```python
from build123d import *

# Parameters (mm, degrees)
PAD002_DEPTH    = 3
SKETCH008_R     = 1.5
SKETCH008_W     = 3
SKETCH008_H     = 26
POCKET001_DEPTH = 3.001
POCKET002_DEPTH = 3.001
SKETCH011_R     = 2.25
HOLE003_DEPTH   = 3.001


with BuildPart() as part:
    # Sketch005 → Pad002 (new body)
    with BuildSketch(Plane.XZ):
        Polygon((-30, 0), (-30, 70), (50, 70), (50, 0), (25, 0), (25, 5.5), (26.5, 5.5), (26.5, 10), (20.5, 10), (20.5, 5.5), (22, 5.5), (22, 0), (20.5, 0), (20.5, -3), (-15.5, -3), (-15.5, 0), (-17, 0), (-17, 5.5), (-15.5, 5.5), (-15.5, 10), (-21.5, 10), (-21.5, 5.5), (-20, 5.5), (-20, 0), align=None)
    extrude(amount=PAD002_DEPTH)

    # Sketch008 (on Face25 of Pad002) → Pocket001 (cut, through all)
    with BuildSketch(Plane(origin=(0, 0, 0), x_dir=(1, 0, 0), z_dir=(0, 1, 0))):
        with Locations((-1.5, -33)):
            Circle(SKETCH008_R)
        with Locations((-1.5, -17)):
            Rectangle(SKETCH008_W, SKETCH008_H)
    extrude(amount=-POCKET001_DEPTH, mode=Mode.SUBTRACT)

    # Sketch009 (on Face4 of Pocket001) → Pocket002 (cut, through all)
    with BuildSketch(Plane(origin=(0, 0, 0), x_dir=(1, 0, 0), z_dir=(0, 1, 0))):
        Polygon((-4, -41), (37, -41), (37, -50.25), (44, -50.25), (44, -52.25), (37.088989, -52.25), (37.088989, -61.5), (-3.911011, -61.5), (-3.911011, -52.25), (-11, -52.25), (-11, -50.25), (-4, -50.25), align=None)
    extrude(amount=-POCKET002_DEPTH, mode=Mode.SUBTRACT)

    # Sketch011 (on Face5 of Pocket002) → Hole003 (cut, through all)
    with BuildSketch(Plane.XZ.offset(3)):
        with Locations((-8, 56.2)):
            Circle(SKETCH011_R)
        with Locations((-8, 46.3)):
            Circle(SKETCH011_R)
        with Locations((40.5, 56.2)):
            Circle(SKETCH011_R)
        with Locations((40.5, 46.3)):
            Circle(SKETCH011_R)
    extrude(amount=-HOLE003_DEPTH, mode=Mode.SUBTRACT)


with BuildPart() as part_1:
    # Body002 placement: moved
    add(part.part.moved(Location((-180, 156, 84))))


solid = part_1.part
```
Can you work these out from the model? Positions are in its coordinate system, mm. A direction names the side the tool comes from. Give positions to 0.01 mm unless a question says otherwise; leave off trailing zeros. Order: outer loops, then holes, each group sorted by start corner. A loop starts at its lowest first (then second) coordinate and runs counter-clockwise, first axis right, second up. Notation, with made-up numbers: M 21,69.25 L 45,69.25 A24 ccw 45,100.25 Z; hole C 2.25,56.25 d7. An arc over 180 degrees is marked long. Write item = value, one per line. Start each with the question number.
Q1. Will these pins go through, and if not, where does the flat tip stop? pin 1 Ø1.6 at (x, y) = (-196.5, 154) entering from -Z; pin 2 Ø1.5 at (y, z) = (154, 82) entering from -X.
Q2. For faces 1 (the flat face through (-188, 155, 134.25)), 2 (the flat face through (-169, 156, 118)), which set-ups out of +Z, -Z, +X, -X, +Y, -Y let a thin tool reach every point of the face, with its end or its side?
Q3. Suppose I cut it at B-B (z = 117). Write out the boundary of the cut face in (x, y), plus the area to 3 significant figures.
Q4. We'd pull the mould along Z, two halves only. Please class faces 3 (the flat face through (-158, 155, 87)), 4 (the flat face through (-183, 155, 101)), 5 (the flat face through (-171, 155, 154)), 6 (the flat face through (-205, 155, 84)): pulls with the +Z half, pulls with the -Z half, needs draft (parallel to the pull), parting line crosses it, or undercut.
Q5. Suppose I cut it at D-D (x = -150). Write out the boundary of the cut face in (y, z).
Q6. Suppose I cut it at A-A (x = -139.5). Write out the boundary of the cut face in (y, z), plus the area to 3 significant figures.
Q7. I need wall thicknesses on probe 1 along Z at (x, y) = (-188, 154); probe 2 along X at (y, z) = (155.6, 89); probe 3 along Z at (x, y) = (-139.5, 155.25). Which ranges of each line are inside material? Lowest first, please. Write a range as [from, to].
Q8. Suppose I cut it at C-C (z = 130.3). Write out the boundary of the cut face in (x, y).
Check result:
q1.pin_1 = 84
q1.pin_2 = -195.5
q2.face_1 = +Y, -Y
q2.face_2 = +Z, -Z, +X, -X, +Y
q3.outline = M -210,153 L -183,153 L -183,156 L -210,156 Z; M -180,153 L -130,153 L -130,156 L -180,156 Z
q3.area = 231 mm2
q4.face_3 = needs draft
q4.face_4 = undercut
q4.face_5 = pulls with the +Z half
q4.face_6 = pulls with the -Z half
q5.outline = M 153,84 L 156,84 L 156,125 L 153,125 Z; M 153,145.5 L 156,145.5 L 156,154 L 153,154 Z
q6.outline = M 153,84 L 156,84 L 156,128.05 L 153,128.05 Z; M 153,132.55 L 156,132.55 L 156,134.25 L 153,134.25 Z; M 153,136.25 L 156,136.25 L 156,137.95 L 153,137.95 Z; M 153,142.45 L 156,142.45 L 156,154 L 153,154 Z
q6.area = 177 mm2
q7.probe_1 = [81, 128.05], [132.55, 134.25], [136.25, 137.95], [142.45, 154]
q7.probe_2 = [-210, -200], [-197, -183], [-180, -158], [-155, -130]
q7.probe_3 = [84, 128.05], [132.55, 134.25], [136.25, 137.95], [142.45, 154]
q8.outline = M -210,153 L -190.25,153 L -190.25,156 L -210,156 Z; M -185.75,153 L -184,153 L -184,156 L -185.75,156 Z; M -143,153 L -141.75,153 L -141.75,156 L -143,156 Z; M -137.25,153 L -130,153 L -130,156 L -137.25,156 Z
